Geometry check sheet. Reference: the model listing, model coordinates, mm. Face numbers are marked on the shaded views. A direction names the side the tool comes from. Round coordinates to 2 decimals unless told otherwise and drop trailing zeros. Order: outer loops, then holes, each group sorted by start corner. A loop starts at its lowest first (then second) coordinate and runs counter-clockwise, first axis right, second up.
(1) Thickness scan on L1, parallel to X at y = 23, z = 0; L2, parallel to X at y = 21.65, z = 0; L3, parallel to Z at x = 5, y = 8. Record the ranges inside material, lowest first.
(2) Gauge pin test, flat ends, axial feed: P1, Ø2, axis at x = -19.5, y = 59, coming from the -Z side; P2, Ø3.5, axis at x = -5.75, z = 0, coming from the +Y side; P3, Ø1.6, axis at y = 23.5, z = -0.5, coming from the +X side. Record the tip position at first contact, or that the pin passes through.
(3) Set-up check for the marked faces 1, 2 and 3: record each of +Z, -Z, +X, -X, +Y, -Y from which the full face is reachable in a straight line by a thin tool's end or side.
(4) Cross-section at B-B on y = 62. Enter the section's corners in (x, z), and give its area (3 significant figures).
(5) Cross-section at D-D on y = 29. Enter the section's corners in (x, z).
(6) Cross-section at C-C on x = -14.5. Enter the section's corners in (y, z), and give its area (3 significant figures).
(7) Draft check along X on the marked faces 4, 5, 6 and 7. Enter one of: pulls with the +X half, pulls with the -X half, needs draft (parallel to the pull), parting line crosses it, or undercut.
(8) Cross-section at A-A on y = 14. Enter the section's corners in (x, z).
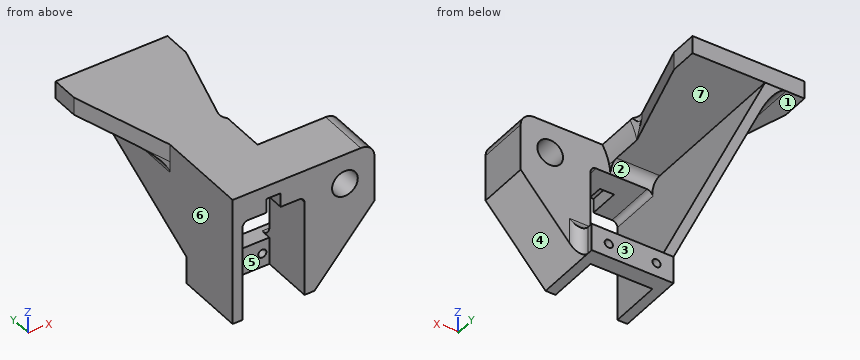
from build123d import *

# Parameters (mm, degrees)
SKETCH2_W            = 30
SKETCH2_H            = 10
BOSS_EXTRUDE1_DEPTH  = 25
SKETCH3_W            = 22.7
SKETCH3_H            = 19
CUT_EXTRUDE1_DEPTH   = 33.388133727
SKETCH4_R            = 1.5
CUT_EXTRUDE2_DEPTH   = 32.208832184
SKETCH5_W            = 3.65
SKETCH5_H            = 19
BOSS_EXTRUDE2_DEPTH  = 37
SKETCH6_W            = 3.65
SKETCH6_H            = 19
BOSS_EXTRUDE3_DEPTH  = 37
SKETCH11_W           = 10
SKETCH11_H           = 19
BOSS_EXTRUDE7_DEPTH  = 22.7
SKETCH12_W           = 5.2
SKETCH12_H           = 5.2
CUT_EXTRUDE4_DEPTH   = 11.1
SKETCH14_W           = 22
SKETCH14_H           = 19
BOSS_EXTRUDE8_DEPTH  = 22
SKETCH15_R           = 4.72
CUT_EXTRUDE6_DEPTH   = 62.032617987
BOSS_EXTRUDE9_DEPTH  = 15
BOSS_EXTRUDE11_DEPTH = 19
BOSS_EXTRUDE12_DEPTH = 6.5
BOSS_EXTRUDE13_DEPTH = 3.65
FILLET1_R            = 5
FILLET2_R            = 4
FILLET3_R            = 2
FILLET5_R            = 4


with BuildPart() as part:
    # Sketch2 → Boss-Extrude1 (new body)
    with BuildSketch(Plane(origin=(0, 0, 0), x_dir=(1, 0, 0), z_dir=(0, 1, 0))):
        with Locations((2.999755729, 0)):
            Rectangle(SKETCH2_W, SKETCH2_H)
    extrude(amount=BOSS_EXTRUDE1_DEPTH)

    # Sketch3 → Cut-Extrude1 (cut, through all)
    with BuildSketch(Plane.XY.offset(5)):
        with Locations((2.999755729, 9.5)):
            Rectangle(SKETCH3_W, SKETCH3_H)
    extrude(amount=-CUT_EXTRUDE1_DEPTH, mode=Mode.SUBTRACT)

    # Sketch4 → Cut-Extrude2 (cut, through all)
    with BuildSketch(Plane.XZ):
        with Locations(Location((-5.750244271, 0, 0), (0, 0, 270))):
            Circle(SKETCH4_R)
        with Locations(Location((11.749755729, 0, 0), (0, 0, 270))):
            Circle(SKETCH4_R)
    extrude(amount=-CUT_EXTRUDE2_DEPTH, mode=Mode.SUBTRACT)

    # Sketch5 → Boss-Extrude2 (add)
    with BuildSketch(Plane.XY.offset(5)):
        with Locations((16.174755729, 9.5)):
            Rectangle(SKETCH5_W, SKETCH5_H)
    extrude(amount=BOSS_EXTRUDE2_DEPTH)

    # Sketch6 → Boss-Extrude3 (add)
    with BuildSketch(Plane.XY.offset(5)):
        with Locations((-10.175244271, 9.5)):
            Rectangle(SKETCH6_W, SKETCH6_H)
    extrude(amount=BOSS_EXTRUDE3_DEPTH)

    # Sketch11 → Boss-Extrude7 (add)
    with BuildSketch(Plane.ZY.offset(-14.349755729)):
        with Locations((37, 9.5)):
            Rectangle(SKETCH11_W, SKETCH11_H)
    extrude(amount=BOSS_EXTRUDE7_DEPTH)

    # Sketch12 → Cut-Extrude4 (cut)
    with BuildSketch(Plane.XZ):
        with Locations((2.999755729, 34.6)):
            Rectangle(SKETCH12_W, SKETCH12_H)
    extrude(amount=-CUT_EXTRUDE4_DEPTH, mode=Mode.SUBTRACT)

    # Sketch14 → Boss-Extrude8 (add)
    with BuildSketch(Plane(origin=(17.999755729, 0, 0), x_dir=(0, 0, -1), z_dir=(1, 0, 0))):
        with Locations((-31, 9.5)):
            Rectangle(SKETCH14_W, SKETCH14_H)
    extrude(amount=BOSS_EXTRUDE8_DEPTH)

    # Sketch15 → Cut-Extrude6 (cut, through all)
    with BuildSketch(Plane(origin=(0, 19, 0), x_dir=(1, 0, 0), z_dir=(0, 1, 0))):
        with Locations(Location((29.179755729, -31, 0), (0, 0, 270))):
            Circle(SKETCH15_R)
    extrude(amount=-CUT_EXTRUDE6_DEPTH, mode=Mode.SUBTRACT)

    # Sketch16 → Boss-Extrude9 (add)
    with BuildSketch(Plane(origin=(0, 19, 0), x_dir=(1, 0, 0), z_dir=(0, 1, 0))):
        with BuildLine():
            Line((-12.000244271, -42), (9.999755729, -42))
            ThreePointArc((9.999755729, -42), (8.508821331, -38.847602891), (7.532067631, -35.5))
            Line((7.532067631, -35.5), (-12.000244271, -35.5))
            Line((-12.000244271, -35.5), (-12.000244271, -42))
        make_face()
    extrude(amount=BOSS_EXTRUDE9_DEPTH)

    # Sketch18 → Boss-Extrude11 (add)
    with BuildSketch(Plane(origin=(0, 19, 0), x_dir=(1, 0, 0), z_dir=(0, 1, 0))):
        Polygon((17.999755729, -20), (17.999755729, 5), (39.999755729, -20), align=None)
    extrude(amount=-BOSS_EXTRUDE11_DEPTH)

    # Sketch19 → Boss-Extrude12 (add)
    with BuildSketch(Plane.XY.offset(42)):
        Polygon((-22.755932023, 80), (18.287755383, 80), (18.287755383, 70), (7.532067631, 34), (-12.000244271, 34), (-22.755932023, 70), align=None)
    extrude(amount=-BOSS_EXTRUDE12_DEPTH)

    # Sketch20 → Boss-Extrude13 (add)
    with BuildSketch(Plane.ZY.offset(12.000244271)):
        Polygon((5, 25), (35.5, 80), (35.5, 19), (5, 19), align=None)
    extrude(amount=-BOSS_EXTRUDE13_DEPTH)

    # Fillet1
    fillet1_edges = [part.edges().sort_by_distance(p)[0] for p in [
        (39.999755729, 9.5, 42),
    ]]
    fillet(fillet1_edges, radius=FILLET1_R)

    # Fillet2
    # the kernel refuses this fillet: 4 mm, written as the material it adds along each edge
    with BuildSketch(Plane(origin=(17.999755729, 19, 5), x_dir=(1, 0, 0), z_dir=(0, 0, -1))) as fillet2_piece_1_section:
        with BuildLine():
            CenterArc((FILLET2_R, -FILLET2_R), FILLET2_R, 90, 90)
            Line((0, -FILLET2_R), (0, 0))
            Line((0, 0), (FILLET2_R, 0))
        make_face()
    fillet2_piece_1 = extrude(amount=20, mode=Mode.PRIVATE)
    fillet2_piece_1 = split(fillet2_piece_1, bisect_by=Plane(origin=(22.959178632, 19, 0.635707845), z_dir=(-0.7507135169227555, 0, 0.6606278948920247)), keep=Keep.TOP, mode=Mode.PRIVATE)
    add(fillet2_piece_1)
    with BuildSketch(Plane(origin=(-12.000244271, 90, 35.5), x_dir=(0, 0, -1), z_dir=(0, -1, 0))) as fillet2_piece_2_section:
        with BuildLine():
            CenterArc((FILLET2_R, -FILLET2_R), FILLET2_R, 90, 90)
            Line((0, -FILLET2_R), (0, 0))
            Line((0, 0), (FILLET2_R, 0))
        make_face()
    fillet2_piece_2 = extrude(amount=66, mode=Mode.PRIVATE)
    fillet2_piece_2 = split(fillet2_piece_2, bisect_by=Plane(origin=(-27.36023555, 85.410909165, 35.5), z_dir=(0.9581502749407442, 0.2862656993615832, 0)), keep=Keep.TOP, mode=Mode.PRIVATE)
    fillet2_piece_2 = split(fillet2_piece_2, bisect_by=Plane(origin=(-12.000244271, 87.648062701, 39.741198407), z_dir=(0, -0.48496776166331645, 0.8745320292289315)), keep=Keep.TOP, mode=Mode.PRIVATE)
    add(fillet2_piece_2)
    with BuildSketch(Plane(origin=(17.999755729, 19, 5), x_dir=(0, 0, 1), z_dir=(-1, 0, 0))) as fillet2_piece_3:
        with BuildLine():
            CenterArc((FILLET2_R, FILLET2_R), FILLET2_R, 180, 90)
            Line((0, FILLET2_R), (0, 0))
            Line((0, 0), (FILLET2_R, 0))
        make_face()
    extrude(amount=3.65)
    with BuildSketch(Plane(origin=(17.453635047, 19, 35.5), x_dir=(0, 0, -1), z_dir=(-1, 0, 0))) as fillet2_piece_4_section:
        with BuildLine():
            CenterArc((4, -3.968626967), FILLET2_R, 97.180755781, 82.819244219)
            Line((0, -3.968626967), (0, 0))
            Line((0, 0), (3.5, 0))
        make_face()
    fillet2_piece_4 = extrude(amount=35.725446735, mode=Mode.PRIVATE)
    fillet2_piece_4 = fillet2_piece_4 - Plane(origin=(29.179755729, 19, 31), x_dir=(-0.8674627670502353, 0, 0.49750210831869773), z_dir=(0, -1, 0)) * Cylinder(22.110459064, 88, mode=Mode.PRIVATE)
    fillet2_piece_4 = split(fillet2_piece_4, bisect_by=Plane(origin=(-12.000244271, 19, 35.5), z_dir=(1, 0, 0)), keep=Keep.TOP, mode=Mode.PRIVATE)
    add(fillet2_piece_4)
    with BuildSketch(Plane(origin=(17.999755729, 19, 15), x_dir=(1, 0, 0), z_dir=(0, 0, -1))) as fillet2_piece_5a_section:
        with BuildLine():
            CenterArc((FILLET2_R, -FILLET2_R), FILLET2_R, 90, 90)
            Line((0, -FILLET2_R), (0, 0))
            Line((0, 0), (FILLET2_R, 0))
        make_face()
    fillet2_piece_5a = extrude(amount=20, mode=Mode.PRIVATE)
    fillet2_piece_5a = split(fillet2_piece_5a, bisect_by=Plane(origin=(17.999755729, 19, 5), z_dir=(0, 0, 1)), keep=Keep.TOP, mode=Mode.PRIVATE)
    with BuildSketch(Plane(origin=(27.999755729, 19, 5), x_dir=(0, 0, 1), z_dir=(-1, 0, 0))) as fillet2_piece_5b_section:
        with BuildLine():
            CenterArc((FILLET2_R, FILLET2_R), FILLET2_R, 180, 90)
            Line((0, FILLET2_R), (0, 0))
            Line((0, 0), (FILLET2_R, 0))
        make_face()
    fillet2_piece_5b = extrude(amount=13.65, mode=Mode.PRIVATE)
    fillet2_piece_5b = split(fillet2_piece_5b, bisect_by=Plane(origin=(27.323470787, 19, 5.595130748), z_dir=(-0.7507135169227555, 0, 0.6606278948920247)), keep=Keep.TOP, mode=Mode.PRIVATE)
    fillet2_piece_5b = split(fillet2_piece_5b, bisect_by=Plane(origin=(17.999755729, 19, 5), z_dir=(1, 0, 0)), keep=Keep.TOP, mode=Mode.PRIVATE)
    fillet2_piece_5 = fillet2_piece_5a & fillet2_piece_5b
    add(fillet2_piece_5)

    # Fillet3
    fillet3_edges = [part.edges().sort_by_distance(p)[0] for p in [
        (14.349755729, 9.5, 32),
        (-8.350244271, 9.5, 32),
    ]]
    fillet(fillet3_edges, radius=FILLET3_R)

    # Fillet5
    # the kernel refuses this fillet: 4 mm, written as the material it adds along each edge
    with BuildSketch(Plane(origin=(7.532067631, 34, 42), x_dir=(0.2862656993615828, 0.9581502749407443, 0), z_dir=(0, 0, -1))) as fillet5_piece_1_section:
        with BuildLine():
            CenterArc((FILLET5_R * 1.34244672574, FILLET5_R), FILLET5_R, 163.365479622, 106.634520378)
            Line((FILLET5_R * 0.3842964508, FILLET5_R * 1.28626569936), (0, 0))
            Line((0, 0), (FILLET5_R * 1.34244672574, 0))
        make_face()
    fillet5_piece_1 = extrude(amount=6.5, mode=Mode.PRIVATE)
    fillet5_piece_1 = fillet5_piece_1 - Plane(origin=(29.179755729, 34, 31), x_dir=(-0.8674627670500467, 0, 0.49750210831902675), z_dir=(0, -1, 0)) * Cylinder(22.110459064, 35, mode=Mode.PRIVATE)
    add(fillet5_piece_1)


solid = part.part
Found:
1. L1: x = -12 to -7.25, -4.25 to 10.25, 13.25 to 18
1. L2: x = -12 to -7.25, -4.25 to 10.25, 13.25 to 18.23
1. L3: z = 37.2 to 42
2. P1: stops at z = 35.5
2. P2: stops at y = 25
2. P3: stops at x = 18.01
3. face 1: -Z, -X, +Y, -Y
3. face 2: +X, +Y
3. face 3: -Z, +X, -X, +Y
4. outline: (-20.37, 35.5) - (-16, 35.5) arc R4 cw to (-12, 31.5) - (-12, 25.52) - (-8.35, 25.52) - (-8.35, 35.5) - (15.9, 35.5) - (15.9, 42) - (-20.37, 42) - close
4. area: 276 mm2
5. outline: (-12, 7.22) - (-8.35, 7.22) - (-8.35, 35.5) - (7.53, 35.5) arc R22.11 cw to (10, 42) - (-12, 42) - close
6. outline: (42.37, 35.21) - (79.47, 35.21) - (80, 35.5) - (80, 42) - (42.37, 42) - close
6. area: 256 mm2
7. face 4: pulls with the +X half
7. face 5: undercut
7. face 6: pulls with the -X half
7. face 7: needs draft
8. outline: (-12, -5) - (-8.35, -5) - (-8.35, 30) arc R2 cw to (-6.35, 32) - (12.35, 32) arc R2 cw to (14.35, 30) - (14.35, -5) - (18, -5) - (40, 20) - (40, 37) arc R5 ccw to (35, 42) - (-12, 42) - close; hole circle Ø9.44 at (29.18, 31)
